Design review of the part built by this model. Coordinates are the model's own, in mm. A direction names the side the tool comes from. Round coordinates to 2 decimals unless told otherwise and drop trailing zeros. Write each loop counter-clockwise with the first axis right and the second up, starting at its lowest first coordinate (ties: lowest second). Pieces come first, ordered by that corner, then holes. Notation, with made-up numbers: M -7,73.5 L 44,73.5 A21 cw 44,80.5 Z; hole C 56.5,42.5 d6. An arc over 180 degrees is marked long. Use CSV: the item, a comma, the result in double quotes.
from build123d import *

# Parameters (mm, degrees)
CROQUIS1_W               = 630
CROQUIS1_H               = 430
CROQUIS1_W_2             = 600
CROQUIS1_H_2             = 400
SALIENTE_EXTRUIR1_DEPTH  = 30
CROQUIS2_R               = 25
SALIENTE_EXTRUIR2_DEPTH  = 40
CROQUIS3_R               = 8
SALIENTE_EXTRUIR3_DEPTH  = 655
CROQUIS4_W               = 24.992302178
CROQUIS4_H               = 432.519106968
SALIENTE_EXTRUIR4_DEPTH  = 30
CROQUIS5_R               = 21.487484315
SALIENTE_EXTRUIR5_DEPTH  = 30
CROQUIS6_W               = 37.188725544
CROQUIS6_H               = 21.959056988
SALIENTE_EXTRUIR6_DEPTH  = 5
CROQUIS7_R               = 25
SALIENTE_EXTRUIR7_DEPTH  = 40
CROQUIS8_R               = 6
SALIENTE_EXTRUIR9_DEPTH  = 470.038213936
CROQUIS9_W               = 23.953368217
CROQUIS9_H               = 15.340921218
SALIENTE_EXTRUIR10_DEPTH = 15
CROQUIS10_W              = 20.266041209
CROQUIS10_H              = 30
SALIENTE_EXTRUIR11_DEPTH = 60
CROQUIS11_R              = 25
SALIENTE_EXTRUIR12_DEPTH = 40
CROQUIS12_W              = 2.6069841
CROQUIS12_H              = 30
SALIENTE_EXTRUIR13_DEPTH = 30
SALIENTE_EXTRUIR14_REACH = 477.248
CROQUIS13_R              = 6
CROQUIS14_W              = 3.214241105
CROQUIS14_H              = 30
SALIENTE_EXTRUIR15_DEPTH = 40
CROQUIS16_R              = 12
SALIENTE_EXTRUIR16_DEPTH = 10
SALIENTE_EXTRUIR16_TAPER = 30
CROQUIS17_R              = 12
SALIENTE_EXTRUIR17_DEPTH = 10
SALIENTE_EXTRUIR17_TAPER = 30
CROQUIS18_R              = 12
SALIENTE_EXTRUIR18_DEPTH = 10
SALIENTE_EXTRUIR18_TAPER = 30
CROQUIS19_R              = 6
CORTAR_EXTRUIR1_DEPTH    = 70


with BuildPart() as part:
    # Croquis1 → Saliente-Extruir1 (new body)
    with BuildSketch(Plane.XY):
        Rectangle(CROQUIS1_W, CROQUIS1_H)
        Rectangle(CROQUIS1_W_2, CROQUIS1_H_2, mode=Mode.SUBTRACT)
    extrude(amount=SALIENTE_EXTRUIR1_DEPTH)

    # Croquis2 → Saliente-Extruir2 (add)
    with BuildSketch(Plane(origin=(315, 0, 0), x_dir=(0, 0, -1), z_dir=(1, 0, 0))):
        with Locations(Location((-15, 0, 0), (0, 0, 233.130102354))):
            Circle(CROQUIS2_R)
    extrude(amount=SALIENTE_EXTRUIR2_DEPTH)

    # Croquis3 → Saliente-Extruir3 (add)
    with BuildSketch(Plane(origin=(355, 0, 0), x_dir=(0, 0, -1), z_dir=(1, 0, 0))):
        with Locations(Location((-15, 0, 0), (0, 0, 180))):
            Circle(CROQUIS3_R)
    extrude(amount=-SALIENTE_EXTRUIR3_DEPTH)

    # Croquis4 → Saliente-Extruir4 (add)
    with BuildSketch(Plane(origin=(0, 0, 0), x_dir=(0, 0, -1), z_dir=(1, 0, 0))):
        with Locations((-42.496151089, -1.259553484)):
            Rectangle(CROQUIS4_W, CROQUIS4_H)
    extrude(amount=SALIENTE_EXTRUIR4_DEPTH)

    # Croquis5 → Saliente-Extruir5 (add)
    with BuildSketch(Plane(origin=(30, 0, 0), x_dir=(0, 0, -1), z_dir=(1, 0, 0))):
        with Locations((-24.875396623, 0)):
            Circle(CROQUIS5_R)
    extrude(amount=-SALIENTE_EXTRUIR5_DEPTH)

    # Croquis6 → Saliente-Extruir6 (add)
    with BuildSketch(Plane.XZ.offset(217.519106968)):
        with Locations((14.477087252, 64.71265509)):
            Rectangle(CROQUIS6_W, CROQUIS6_H)
    saliente_extruir6 = extrude(amount=-SALIENTE_EXTRUIR6_DEPTH)

    # Simetría1: Saliente-Extruir6 across plane
    add(saliente_extruir6.mirror(Plane.ZX))

    # Croquis7 → Saliente-Extruir7 (add)
    with BuildSketch(Plane.XZ.offset(217.519106968)):
        with Locations(Location((14.477087252, 64.71265509, 0), (0, 0, 308.383093816))):
            Circle(CROQUIS7_R)
    extrude(amount=SALIENTE_EXTRUIR7_DEPTH)

    # Croquis8 → Saliente-Extruir9 (add)
    with BuildSketch(Plane.XZ.offset(257.519106968)):
        with Locations(Location((14.477087252, 64.71265509, 0), (0, 0, 270))):
            Circle(CROQUIS8_R)
    extrude(amount=-SALIENTE_EXTRUIR9_DEPTH)

    # Croquis9 → Saliente-Extruir10 (add, symmetric)
    with BuildSketch(Plane(origin=(0, 0, 0), x_dir=(1, 0, 0), z_dir=(0, 1, 0))):
        with Locations((14.702855752, -65.412295985)):
            Rectangle(CROQUIS9_W, CROQUIS9_H)
    extrude(amount=SALIENTE_EXTRUIR10_DEPTH, both=True)

    # Croquis10 → Saliente-Extruir11 (add)
    with BuildSketch(Plane.XY.offset(73.082756594)):
        with Locations((12.859192248, 0)):
            Rectangle(CROQUIS10_W, CROQUIS10_H)
    extrude(amount=SALIENTE_EXTRUIR11_DEPTH)

    # Croquis11 → Saliente-Extruir12 (add)
    with BuildSketch(Plane.XY.offset(133.082756594)):
        with Locations(Location((30, 0, 0), (0, 0, 216.869897646))):
            Circle(CROQUIS11_R)
    extrude(amount=SALIENTE_EXTRUIR12_DEPTH)

    # Croquis12 → Saliente-Extruir13 (add)
    with BuildSketch(Plane(origin=(26.67953986, 0, 0), x_dir=(0, 0, -1), z_dir=(1, 0, 0))):
        with Locations((-59.045327426, 0)):
            Rectangle(CROQUIS12_W, CROQUIS12_H)
    extrude(amount=SALIENTE_EXTRUIR13_DEPTH)

    # Saliente-Extruir14: up to this face of the body (flat: up to its plane)
    saliente_extruir14_end = Plane(part.part.faces().sort_by_distance((41.67953986, 0, 60.348819476))[0])
    # Croquis13 → Saliente-Extruir14 (add, up to the picked face)
    with BuildSketch(Plane.XY.offset(173.082756594), mode=Mode.PRIVATE) as saliente_extruir14_sk1:
        with Locations((30, 0)):
            Circle(CROQUIS13_R)
    saliente_extruir14_tool1 = split(extrude(saliente_extruir14_sk1.sketch, amount=-SALIENTE_EXTRUIR14_REACH, mode=Mode.PRIVATE), bisect_by=saliente_extruir14_end, keep=Keep.BOTH, mode=Mode.PRIVATE)
    add(saliente_extruir14_tool1.solids().sort_by(Axis((30, 0, 173.082757), (0, 0, -1)))[0])

    # Croquis14 → Saliente-Extruir15 (add)
    with BuildSketch(Plane(origin=(22.992212852, 0, 0), x_dir=(0, 0, -1), z_dir=(1, 0, 0))):
        with Locations((-131.475636042, 0)):
            Rectangle(CROQUIS14_W, CROQUIS14_H)
    extrude(amount=SALIENTE_EXTRUIR15_DEPTH)

    # Croquis16 → Saliente-Extruir16 (add)
    with BuildSketch(Plane(origin=(355, 0, 0), x_dir=(0, 0, -1), z_dir=(1, 0, 0))):
        with Locations((-15, 0)):
            Circle(CROQUIS16_R)
    extrude(amount=SALIENTE_EXTRUIR16_DEPTH, taper=SALIENTE_EXTRUIR16_TAPER)

    # Croquis17 → Saliente-Extruir17 (add)
    with BuildSketch(Plane.XZ.offset(257.519106968)):
        with Locations((14.477087252, 64.71265509)):
            Circle(CROQUIS17_R)
    extrude(amount=SALIENTE_EXTRUIR17_DEPTH, taper=SALIENTE_EXTRUIR17_TAPER)

    # Croquis18 → Saliente-Extruir18 (add)
    with BuildSketch(Plane.XY.offset(173.082756594)):
        with Locations((29.930352353, 0)):
            Circle(CROQUIS18_R)
    extrude(amount=SALIENTE_EXTRUIR18_DEPTH, taper=SALIENTE_EXTRUIR18_TAPER)

    # Croquis19 → Cortar-Extruir1 (cut)
    with BuildSketch(Plane(origin=(30, 0, 0), x_dir=(0, 0, -1), z_dir=(1, 0, 0))):
        with Locations((-43.031639772, -205.41246119)):
            Circle(CROQUIS19_R)
        with Locations((-43.031639772, -179.41246119)):
            Circle(CROQUIS19_R)
        with Locations((-43.031639772, -153.41246119)):
            Circle(CROQUIS19_R)
        with Locations((-43.031639772, -127.41246119)):
            Circle(CROQUIS19_R)
        with Locations((-43.031639772, -101.41246119)):
            Circle(CROQUIS19_R)
        with Locations((-43.031639772, -75.41246119)):
            Circle(CROQUIS19_R)
        with Locations((-43.031639772, -49.41246119)):
            Circle(CROQUIS19_R)
        with Locations((-43.031639772, -23.41246119)):
            Circle(CROQUIS19_R)
        with Locations((-43.031639772, 2.58753881)):
            Circle(CROQUIS19_R)
        with Locations((-43.031639772, 28.58753881)):
            Circle(CROQUIS19_R)
        with Locations((-43.031639772, 54.58753881)):
            Circle(CROQUIS19_R)
        with Locations((-43.031639772, 80.58753881)):
            Circle(CROQUIS19_R)
        with Locations((-43.031639772, 106.58753881)):
            Circle(CROQUIS19_R)
        with Locations((-43.031639772, 132.58753881)):
            Circle(CROQUIS19_R)
        with Locations((-43.031639772, 158.58753881)):
            Circle(CROQUIS19_R)
        with Locations((-43.031639772, 184.58753881)):
            Circle(CROQUIS19_R)
    extrude(amount=-CORTAR_EXTRUIR1_DEPTH, mode=Mode.SUBTRACT)


solid = part.part
1) Add section A-A on z = 118.5. Write out the cut boundary in (x, y), then the cut area to 3 significant figures.
Answers:
outline,"M 2.73,-15 L 22.99,-15 L 22.99,15 L 2.73,15 Z; C 30,0 d12"
area,"721 mm²"
2) Add section C-C on z = 161. Write out the cut boundary in (x, y), then the cut area to 3 significant figures.
Answers:
outline,"C 30,0 d50"
area,"1,960 mm²"
3) Machinability: for faces 4 (the face through (-147.9, 4.868, 8.651)), 5 (the face through (41, 6, 173.083)), 6 (the face through (20.4, -257.519, 54)), which of the approach directions +Z, -Z, +X, -X, +Y, -Y give a long, thin tool a straight path to every point of the face, cutting with its end or side? Answer none if there is none.
Answers:
face 4,"none"
face 5,"+Z"
face 6,"-Y"
4) For pin 1 Ø15 at (x, y) = (17, 154) entering from -Z; pin 2 Ø15 at (y, z) = (-127.5, 11.5) entering from +X; pin 3 Ø15.5 at (y, z) = (-179.41, 43.03) entering from -X, all flat-tipped, find the tip position at first contact; note any pin that passes through.
Answers:
pin 1,"z = 30"
pin 2,"x = 315"
pin 3,"x = 0"
5) Wall thickness on line 1 along Y through (x, z) = (-160, 6.5); line 2 along X through (y, z) = (-160, 29); line 3 along Y through (x, z) = (-49, 18): over which ranges is each line inside the solid? List them lowest first. Write a range as [from, to].
Answers:
line 1,"[-215, -200], [200, 215]"
line 2,"[-315, -300], [300, 315]"
line 3,"[-215, -200], [-7.42, 7.42], [200, 215]"
6) The part is to be moulded in two halves that separate along Z. For faces 1 (the face through (13.63, -267.034, 71.164)), 2 (the face through (-300, -3, 25)), 3 (the face through (43, 0, 129.869)), say which applies: released by +Z, released by -Z, zero draft, split by the parting line, or undercut.
Answers:
face 1,"split by the parting line"
face 2,"zero draft"
face 3,"undercut"
7) Add section B-B on x = 208.5. Write out the cut boundary in (y, z).
Answers:
outline,"M -215,0 L -200,0 L -200,30 L -215,30 Z; C 0,15 d16; M 200,0 L 215,0 L 215,30 L 200,30 Z"
